Autodesk Inventor part; units mm, degrees
ref_plane "YZ Plane" through (0, 0, 0) normal (1, 0, 0) x (0, 1, 0)
ref_plane "XZ Plane" through (0, 0, 0) normal (0, 1, 0) x (-1, 0, 0)
ref_plane "XY Plane" through (0, 0, 0) normal (0, 0, 1) x (1, 0, 0)
sketch "Sketch1" plane through (0, 0, 0) normal (0, 0, 1) x (1, 0, 0)
  circle A0 centre (0, 30) radius 8.45 construction
  circle A1 centre (0, 30) radius 3.5
  arc A2 (-30, 0) -> (-15.2201, 12.4401) centre (-30, 15) ccw
  arc A3 (15.2201, 12.4401) -> (30, 0) centre (30, 15) ccw
  arc A4 (11.824, 32.0479) -> (-11.824, 32.0479) centre (0, 30) ccw
  line L0 (-11.824, 32.0479) -> (-15.2201, 12.4401)
  line L1 (11.824, 32.0479) -> (15.2201, 12.4401)
  line L2 (30, 0) -> (-30, 0)
  line L3 (-30, 0) -> (-30, -2.5)
  line L4 (-30, -2.5) -> (30, -2.5)
  line L5 (30, -2.5) -> (30, 0)
  point P0 (0, 0)
  point P1 (0, 0)
  point P2 (0, 0)
  dimension "d0" = 16.9
  dimension "d1" = 7
  dimension "d2" = 30
  dimension "d3" = 12
  dimension "d4" = 15
  dimension "d5" = 60
  dimension "d6" = 2.5
extrude "Extrusion1" add sketch "Sketch1" along normal blind 20 contours A1 | A2 L0 A4 L1 A3 L2
extrude "Extrusion3" add sketch "Sketch1" along normal blind 20 contours L2 L5 L4 L3
ref_plane "Work Plane1" through (-30, -2.5, 0) normal (0, -1, 0) x (1, 0, 0)
sketch "Sketch2" plane through (-30, -2.5, 0) normal (0, -1, 0) x (1, 0, 0)
  line L0 (21.55, 20) -> (38.45, 20)
  line L1 (30, 20) -> (30, 60) construction
  line L2 (60, 0) -> (60, 20) construction
  line L3 (30, 20) -> (52.9431, 52.7661) construction
  line L4 (47.9062, 63.0072) -> (64.2892, 51.5357)
  line L5 (64.2892, 51.5357) -> (61.1346, 47.0303)
  line L6 (61.1346, 47.0303) -> (44.7515, 58.5018) construction
  line L7 (44.7515, 58.5018) -> (47.9062, 63.0072)
  line L8 (44.7515, 58.5018) -> (17.7923, 20)
  line L9 (41.824, 20) -> (18.176, 20)
  line L10 (61.1346, 47.0303) -> (42.2077, 20)
  line L11 (0, 20) -> (60, 20)
  point P0 (30, 0)
  dimension "d14" = 35
  dimension "d16" = 5.5
  dimension "d17" = 20
  dimension "d26" = 40
extrude "Extrusion6" add sketch "Sketch2" against normal blind 2.5
sketch "Sketch4" plane through (34.2892, -2.5, 51.5357) normal (0.5735764, 0, 0.819152) x (0.819152, 0, -0.5735764)
  line L0 (-23.103, 0) -> (-34.5746, 0)
  circle A0 centre (-10, 10.5) radius 7.3 construction
  circle A1 centre (-10, 10.5) radius 5.35
  line L1 (-16.2022, 2.5) -> (-3.7978, 2.5)
  line L2 (-3.7978, 2.5) -> (-3.7978, 6.65)
  line L3 (-3.7978, 6.65) -> (-16.2022, 6.65)
  line L4 (-16.2022, 6.65) -> (-16.2022, 2.5)
  line L5 (-20, 2.5) -> (0, 2.5)
  line L6 (-16.2022, 2.5) -> (-16.2022, 0)
  line L7 (-3.7978, 2.5) -> (-3.7978, 0)
  line L8 (-23.103, 0) -> (26.0461, 0)
  line L9 (0, 0) -> (-20, 0)
  line L10 (0, 0) -> (0, 2.5)
  line L11 (-20, 2.5) -> (0, 2.5)
  line L12 (-20, 0) -> (-20, 2.5)
  point P0 (1.4715, 2.5)
  point P1 (-10, 2.5)
  point P2 (-6.2852, 6.65)
  point P3 (-13.7148, 6.65)
  point P4 (0, 0)
  point P5 (0, 2.5)
  point P6 (-20, 2.5)
  point P7 (-20, 0)
  point P8 (-16.2022, 2.5)
  dimension "d29" = 14.6
  dimension "d30" = 10.7
  dimension "d31" = 1.5
  dimension "d32" = 8
extrude "Extrusion7" add sketch "Sketch4" against normal blind 5.5 contours A1 L3 L2 L1 L4
extrude "Extrusion8" cut sketch "Sketch4" against normal up to surface contours L6 L8 L12 L5 | L5 L10 L8 L7 surface through (0, 21, 20) normal (0, 0, 1)
extrude "Extrusion9" add sketch "Sketch4" along normal blind 7.5 contours L1 L7 L8 L6
extrude "Extrusion10" cut sketch "Sketch1" along normal through all contours A1
properties part number "Support 2 - V1"
Verification items for the finished model (mm, model axes). A direction names the side the tool comes from. Give positions to 0.01 mm unless a question says otherwise; leave off trailing zeros. Order: outer loops, then holes, each group sorted by start corner. A loop starts at its lowest first (then second) coordinate and runs counter-clockwise, first axis right, second up. Notation, with made-up numbers: M 56,17 L 96,17 A7 cw 96,27 Z; hole C 63.25,55 d11. An arc over 180 degrees is marked long. Answer as a JSON object with one key per item and string values. Group by question number.
1) Scan lines: line 1 along Y through (x, z) = (0, 16); line 2 along Z through (x, y) = (6, 28.5); line 3 along Y through (x, z) = (26.5, 62.5). Record each from-to range of solid material in increasing order. Write a range as [from, to].
2) Cross-section at C-C (y = 30). Enter the section's corners in (x, z).
3) Cross-section at D-D (x = -21). Enter the section's corners in (y, z).
4) Access from +Z, -Z, +X, -X, +Y, -Y to the whole of each face (thin tool, end or side, straight path). Record for faces 4 (the face through (20, 4.15, 58)), 5 (the face through (20.454, 3.43, 9.86)), 6 (the face through (28, 0, 60)), 7 (the face through (30, -1, 10)), 8 (the face through (22.872, 1.643, 52.816)).
5) Cross-section at A-A (z = 11). Enter the section's corners in (x, y), then the cut area to 3 significant figures.
6) Mould release check, pull along Z, two halves, no side actions. Record for faces 1 (the face through (0, 15, 0)), 2 (the face through (10, 0, 38)), 3 (the face through (26.03, 1.64, 57.32)): released by +Z, released by -Z, zero draft, split by the parting line, or undercut.
7) Cross-section at B-B (x = 0). Enter the section's corners in (y, z).
8) Depth check by flat-ended pin: pin 1 Ø1.6 at (x, z) = (21, 57.5) entering from +Y; pin 2 Ø2 at (x, y) = (-20.5, 7.5) entering from -Z; pin 3 Ø18 at (x, z) = (11, 32.5) entering from +Y; pin 4 Ø12 at (x, y) = (-19.5, 14.5) entering from +Z. Enter the tip coordinate at first touch or a pass-through.
Result sheet:
{
 "1": {"line 1": "y = [-2.5, 26.5], [33.5, 42]", "line 2": "z = [0, 20]", "line 3": "y = [-2.5, 0]"},
 "2": {"outline": "M -12.18,0 L -3.5,0 L -3.5,20 L -12.18,20 Z; M 3.5,0 L 12.18,0 L 12.18,20 L 3.5,20 Z"},
 "3": {"outline": "M -2.5,0 L 3,0 L 3,20 L -2.5,20 Z"},
 "4": {"face 4": "+Z, +X, -X, +Y", "face 5": "-Z, +X, +Y", "face 6": "+Z, +X, +Y", "face 7": "-Z, +X, +Y, -Y", "face 8": "-X, +Y"},
 "5": {"outline": "M -30,-2.5 L 30,-2.5 L 30,0 A15 cw 15.22,12.44 L 11.82,32.05 A12 ccw -11.82,32.05 L -15.22,12.44 A15 cw -30,0 Z; hole C 0,30 d7", "area": "1,290 mm2"},
 "6": {"face 1": "released by -Z", "face 2": "undercut", "face 3": "released by +Z"},
 "7": {"outline": "M -2.5,0 L 26.5,0 L 26.5,20 L 0,20 L 0,30.81 L -2.5,30.81 Z; M 33.5,0 L 42,0 L 42,20 L 33.5,20 Z"},
 "8": {"pin 1": "stops at y = 4.15", "pin 2": "passes through", "pin 3": "stops at y = 0", "pin 4": "stops at z = 20"}
}
